Source: CAD feature listing. Evaluate the final solid. Frame: model axes, mm. Face numbers are marked on the shaded views. A direction names the side the tool comes from. Give positions to 0.01 mm unless a question says otherwise; leave off trailing zeros. Order: outer loops, then holes, each group sorted by start corner. A loop starts at its lowest first (then second) coordinate and runs counter-clockwise, first axis right, second up. Notation, with made-up numbers: M -38.75,62.5 L 8.25,62.5 A30 ccw 8.25,95.5 Z; hole C -1,84 d1. An arc over 180 degrees is marked long. Use CSV: the item, a comma, the result in double quotes. Start each with the question number.
1. Section query D-D, the plane x = 1. Return the cut outline in (y, z).
2. Reachability of the marked faces 1, 2 and 3 from +Z, -Z, +X, -X, +Y, -Y: full face, straight path, thin tool, end or side. Return the list, or none.
3. Section query C-C, the plane x = -11.25. Return the cut outline in (y, z), plus the area to 3 significant figures.
4. Line query: line 1 along Z through (x, y) = (-1.8, 0); line 2 along Y through (x, z) = (-0.75, -2.5); line 3 along Y through (x, z) = (-1.5, -6.5). Output: solid intervals per line, ascending. Write a range as [from, to].
5. Pin query (flat end, axial travel): P1, Ø3, axis at y = -15.5, z = -7.5, coming from the -X side (3 decimals); P2, Ø1.7, axis at x = 0, z = -0.5, coming from the +Y side; P3, Ø8, axis at x = 0, z = 8.5, coming from the +Y side; P4, Ø1, axis at x = -6, z = -3, coming from the +Y side. Return the tip coordinate at first contact, or that it passes through.
6. Mould query, pull axis Z, two halves, no side actions, for the marked faces 4, 5 and 6. Classes: released by +Z, released by -Z, zero draft, split by the parting line, or undercut.
7. Section query A-A, the plane x = -1.75. State how many separate pieces and enclosed holes the cut face has, plus the area to 3 significant figures.
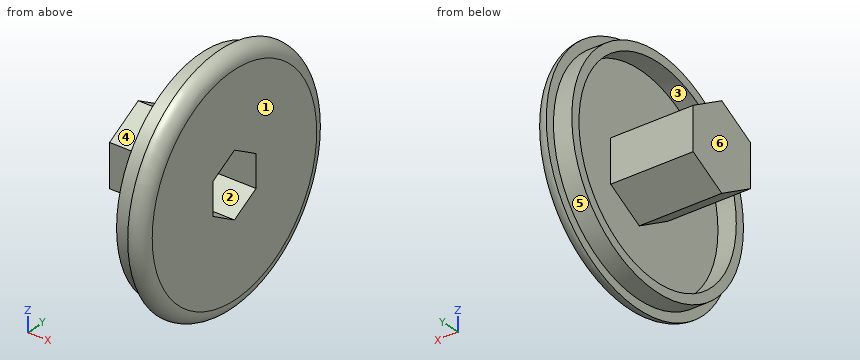
from build123d import *

# Parameters (mm, degrees)
F1_DEPTH = 14.2875
F2_R     = 20.6375
F3_DEPTH = 2.38125
F5_DEPTH = 9.525
F6_R     = 19.05
F6_R_2   = 17.4625
F7_DEPTH = 3.175
F8_R     = 2.38124


# Not quite as in the source:
# - a fillet or chamfer is up to 0.001 mm smaller than in the source, because OpenCascade refuses the exact size


with BuildPart() as f1:
    # F0 (on Right) → F1 (new body)
    with BuildSketch(Plane.YZ):
        Polygon((6.35, -3.6661742094), (6.35, 3.6661742094), (0, 7.3323484187), (-6.35, 3.6661742094), (-6.35, -3.6661742094), (0, -7.3323484187), align=None)
    extrude(amount=-F1_DEPTH)

    # F2 (on Right) → F3 (join)
    with BuildSketch(Plane.YZ):
        Circle(F2_R)
    extrude(amount=F3_DEPTH)

    # F4 (on face) → F5 (cut)
    with BuildSketch(Plane.YZ.offset(2.38125)):
        Polygon((4.7879, -2.7642953539), (4.7879, 2.7642953539), (0, 5.5285907077), (-4.7879, 2.7642953539), (-4.7879, -2.7642953539), (0, -5.5285907077), align=None)
    extrude(amount=-F5_DEPTH, mode=Mode.SUBTRACT)

    # F6 (on face) → F7 (join)
    with BuildSketch(Plane(origin=(0, 0, 0), x_dir=(0, -1, 0), z_dir=(-1, 0, 0))):
        Circle(F6_R)
        Circle(F6_R_2, mode=Mode.SUBTRACT)
    extrude(amount=F7_DEPTH)

    # F8 (radius 2.38125 in the source; OpenCascade refuses exactly that, so slightly less here)
    f8_edges = [f1.edges().sort_by_distance(p)[0] for p in [
        (2.38125, -20.6375, 0),
    ]]
    fillet(f8_edges, radius=F8_R)


solid = f1.part
Result set:
1,outline,"C 0,0 d40.83; hole M -4.79,-2.76 L 0,-5.53 L 4.79,-2.76 L 4.79,2.76 L 0,5.53 L -4.79,2.76 Z"
2,face 1,"+Z, -Z, +X, +Y, -Y"
2,face 2,"+X"
2,face 3,"-X"
3,outline,"M -6.35,-3.67 L 0,-7.33 L 6.35,-3.67 L 6.35,3.67 L 0,7.33 L -6.35,3.67 Z"
3,area,"140 mm2"
4,line 1,"[-19.05, -17.46], [-7.33, -5.53], [5.53, 7.33], [17.46, 19.05]"
4,line 2,"[-18.89, -17.28], [-6.35, -4.79], [4.79, 6.35], [17.28, 18.89]"
4,line 3,"[-17.91, -16.21], [-1.44, 1.44], [16.21, 17.91]"
5,P1,"x = -3.175"
5,P2,"y = 20.64"
5,P3,"y = 20.14"
5,P4,"y = 6.35"
6,face 4,"undercut"
6,face 5,"split by the parting line"
6,face 6,"zero draft"
7,separate pieces,"2"
7,enclosed holes,"2"
7,area,"242 mm2"
